Can you work these out from the model? Positions are in its coordinate system, mm. Round coordinates to 2 decimals unless told otherwise and drop trailing zeros. Loops run counter-clockwise (first coordinate to the right, second up) from the corner with the lowest first, then second, coordinate; pieces in that order, holes last. Notation, with made-up numbers: (53, 9) -> (68, 9) arc R13 cw to (68, 21) -> close; hole circle Ø1 at (-8.75, 35.25). An arc over 180 degrees is marked (long way). Write each question's results on one line, items separated by ' | '.
Autodesk Inventor part; units mm, degrees
ref_plane "YZ Plane" through (0, 0, 0) normal (1, 0, 0) x (0, 1, 0)
ref_plane "XZ Plane" through (0, 0, 0) normal (0, 1, 0) x (-1, 0, 0)
ref_plane "XY Plane" through (0, 0, 0) normal (0, 0, 1) x (1, 0, 0)
sketch "Sketch66" plane through (0, 0, 0) normal (0, 0, 1) x (1, 0, 0)
  line L0 (-10, -10) -> (10, -10)
  line L1 (10, -10) -> (10, 10)
  line L2 (10, 10) -> (-10, 10)
  line L3 (-10, 10) -> (-10, -10)
  line L4 (-10, -10) -> (10, 10) construction
  line L5 (10, -10) -> (-10, 10) construction
  point P0 (0, 0)
  dimension "d179" = 20
  dimension "d180" = 20
extrude "Extrusion45" add sketch "Sketch66" along normal blind 3
sketch "Sketch67" plane through (0, 0, 3) normal (0, 0, 1) x (1, 0, 0)
  circle A0 centre (0, 0) radius 3
  dimension "d183" = 6
extrude "Extrusion46" cut sketch "Sketch67" against normal blind 3
properties part number "magnet_test_print_v2"
1. If we section it at B-B (x = -1): List the corners of the cut face in (y, z) for me.
Final values:
outline: (-10, 0) -> (-2.83, 0) -> (-2.83, 3) -> (-10, 3) -> close; (2.83, 0) -> (10, 0) -> (10, 3) -> (2.83, 3) -> close
2. Will this pin go through, and if not, where does the flat tip stop? pin 1 (5 mm diameter, centred on x = 0, y = 0, fed in from +Z).
Final values:
pin 1: through
3. Please list where these lines run through material, in increasing order: line 1 (Y direction, x = 0, z = 2.15); line 2 (Y direction, x = -2.5, z = 0.7); line 3 (X direction, y = 0.25, z = 2). Write a range as from..to.
Final values:
line 1: -10..-3, 3..10 | line 2: -10..-1.66, 1.66..10 | line 3: -10..-2.99, 2.99..10
4. If we section it at C-C (z = 2.6): List the corners of the cut face in (x, y) for me, then the cut area to 3 significant figures.
Final values:
outline: (-10, -10) -> (10, -10) -> (10, 10) -> (-10, 10) -> close; hole circle Ø6 at (0, 0) | area: 372 mm2
5. If we section it at A-A (y = 0): List the corners of the cut face in (x, z) for me.
Final values:
outline: (-10, 0) -> (-3, 0) -> (-3, 3) -> (-10, 3) -> close; (3, 0) -> (10, 0) -> (10, 3) -> (3, 3) -> close
